from build123d import *

# Parameters (mm, degrees)
BOSS_EXTRUDE1_DEPTH = 60
BOSS_EXTRUDE2_DEPTH = 15
SKETCH3_R           = 16.002353199
SKETCH3_R_2         = 11
BOSS_EXTRUDE3_DEPTH = 20
BOSS_EXTRUDE4_START = 5
SKETCH4_R           = 16
SKETCH4_R_2         = 11
BOSS_EXTRUDE4_DEPTH = 5
SKETCH5_R           = 11
CUT_EXTRUDE2_DEPTH  = 157.074401446
SKETCH6_R           = 8.5
CUT_EXTRUDE3_DEPTH  = 154.528935617


with BuildPart() as part:
    # Sketch1 → Boss-Extrude1 (new body)
    with BuildSketch(Plane(origin=(0, 0, 0), x_dir=(0, 0, -1), z_dir=(1, 0, 0))):
        Polygon((-29.344624104, 0), (-29.344624104, 18), (45.655375896, 18), (45.655375896, -12), (25.655375896, -12), (25.655375896, 0), align=None)
    extrude(amount=-BOSS_EXTRUDE1_DEPTH)

    # Sketch2 → Boss-Extrude2 (add)
    with BuildSketch(Plane.ZY.offset(60)):
        with BuildLine():
            Line((-45.655375896, 18), (29.344624104, 18))
            Line((29.344624104, 18), (-65.655375896, 58))
            Line((-65.655375896, 58), (-89.536995268, 86.31551376))
            ThreePointArc((-89.536995268, 86.31551376), (-113.623611479, 86.744179795), (-110.833026428, 62.815923064))
            Line((-110.833026428, 62.815923064), (-45.655375896, 18))
        make_face()
    extrude(amount=-BOSS_EXTRUDE2_DEPTH)

    # Sketch3 → Boss-Extrude3 (add)
    with BuildSketch(Plane(origin=(-45, 0, 0), x_dir=(0, 0, -1), z_dir=(1, 0, 0))):
        with Locations(Location((101.767701538, 76, 0), (0, 0, 140.837952037))):
            Circle(SKETCH3_R)
        with Locations((101.767701538, 76)):
            Circle(SKETCH3_R_2, mode=Mode.SUBTRACT)
    extrude(amount=BOSS_EXTRUDE3_DEPTH)

    # Sketch4 → Boss-Extrude4 (add)
    with BuildSketch(Plane.ZY.offset(60).offset(BOSS_EXTRUDE4_START)):
        with Locations((-101.767701538, 76)):
            Circle(SKETCH4_R)
        with Locations(Location((-101.767701538, 76, 0), (0, 0, 180))):
            Circle(SKETCH4_R_2, mode=Mode.SUBTRACT)
    extrude(amount=-BOSS_EXTRUDE4_DEPTH)

    # Sketch5 → Cut-Extrude2 (cut, through all)
    with BuildSketch(Plane(origin=(-45, 0, 0), x_dir=(0, 0, -1), z_dir=(1, 0, 0))):
        with Locations(Location((101.767701538, 76, 0), (0, 0, 180))):
            Circle(SKETCH5_R)
    extrude(amount=-CUT_EXTRUDE2_DEPTH, mode=Mode.SUBTRACT)

    # Sketch6 → Cut-Extrude3 (cut, through all)
    with BuildSketch(Plane(origin=(0, 18, 0), x_dir=(1, 0, 0), z_dir=(0, 1, 0))):
        with Locations(Location((-25, -17.344624104, 0), (0, 0, 270))):
            Circle(SKETCH6_R)
        with Locations(Location((-25, 7.655375896, 0), (0, 0, 270))):
            Circle(SKETCH6_R)
    extrude(amount=-CUT_EXTRUDE3_DEPTH, mode=Mode.SUBTRACT)


solid = part.part
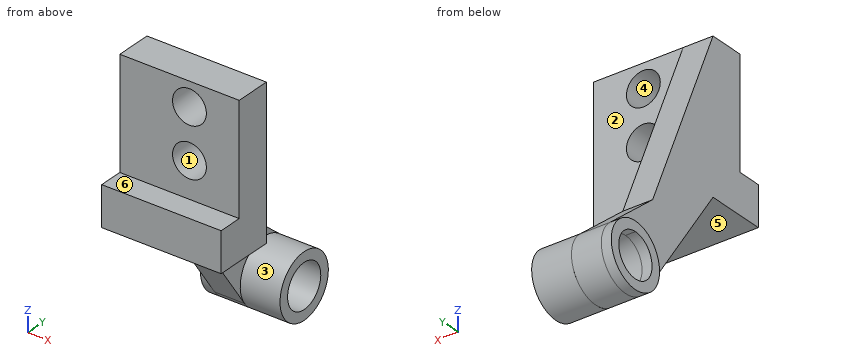
Design review of the part built by this model. Coordinates are the model's own, in mm. Face numbers are marked on the shaded views. A direction names the side the tool comes from. Give positions to 0.01 mm unless a question says otherwise; leave off trailing zeros. Write each loop counter-clockwise with the first axis right and the second up, starting at its lowest first coordinate (ties: lowest second). Pieces come first, ordered by that corner, then holes. Notation, with made-up numbers: M 71.5,-6.5 L 98.5,-6.5 A20 cw 98.5,23.5 Z; hole C -29,62.5 d3. An arc over 180 degrees is marked long. Answer as a JSON object with one key per item and string values. Group by question number.
1) Mouldability with a two-part tool opening along Z and no side actions: class the marked faces 1, 2 and 3 as released by +Z, released by -Z, zero draft, split by the parting line, or undercut.
2) We need section B-B (y = 10). Give the boundary of the cut face in (x, z).
3) We need section A-A (x = -53). Give the boundary of the cut face in (y, z).
4) Tool access review of the marked faces 4, 5 and 6: name each direction out of +Z, -Z, +X, -X, +Y, -Y from which nothing blocks a thin tool from reaching the whole face with its end or side.
5) Clearance check with flat-ended pins moving along their axes: pin 1 Ø9.5 at (x, y) = (-19, -8.5) entering from +Z; pin 2 Ø16 at (y, z) = (76.5, -108.5) entering from +X; pin 3 Ø5 at (x, z) = (-48, -77.5) entering from +Y; pin 4 Ø15.5 at (x, z) = (-25, 17.34) entering from +Y. State where each tip first meets the part, or that it passes through.
6) For line 1 along X through (y, z) = (65, -108); line 2 along X through (y, z) = (46, -47.5); line 3 along Z through (x, y) = (-31, 76), list the stretches that pass through material, from the lowest coordinate up.
7) We need section D-D (x = -11). Give the boundary of the cut face in (y, z), and give its area (3 significant figures).
Answer key:
{
 "1": {"face 1": "undercut", "face 2": "zero draft", "face 3": "split by the parting line"},
 "2": {"outline": "M -60,-45.66 L 0,-45.66 L 0,29.34 L -60,29.34 Z; hole C -25,-7.66 d17; hole C -25,17.34 d17"},
 "3": {"outline": "M -12,-45.66 L 18,-45.66 L 62.82,-110.83 A16 ccw long 86.32,-89.54 L 58,-65.66 L 18,29.34 L 0,29.34 L 0,-25.66 L -12,-25.66 Z; hole C 76,-101.77 d22"},
 "4": {"face 4": "+Y, -Y", "face 5": "-Z, +X, -X, -Y", "face 6": "+Z, +X, -X, -Y"},
 "5": {"pin 1": "stops at z = -25.66", "pin 2": "stops at x = -25", "pin 3": "stops at y = 75.01", "pin 4": "passes through"},
 "6": {"line 1": "x = -65 to -25", "line 2": "x = -60 to -45", "line 3": "z = -117.77 to -112.77, -90.77 to -85.77"},
 "7": {"outline": "M -12,-45.66 L 18,-45.66 L 18,29.34 L 0,29.34 L 0,-25.66 L -12,-25.66 Z", "area": "1,590 mm²"}
}
